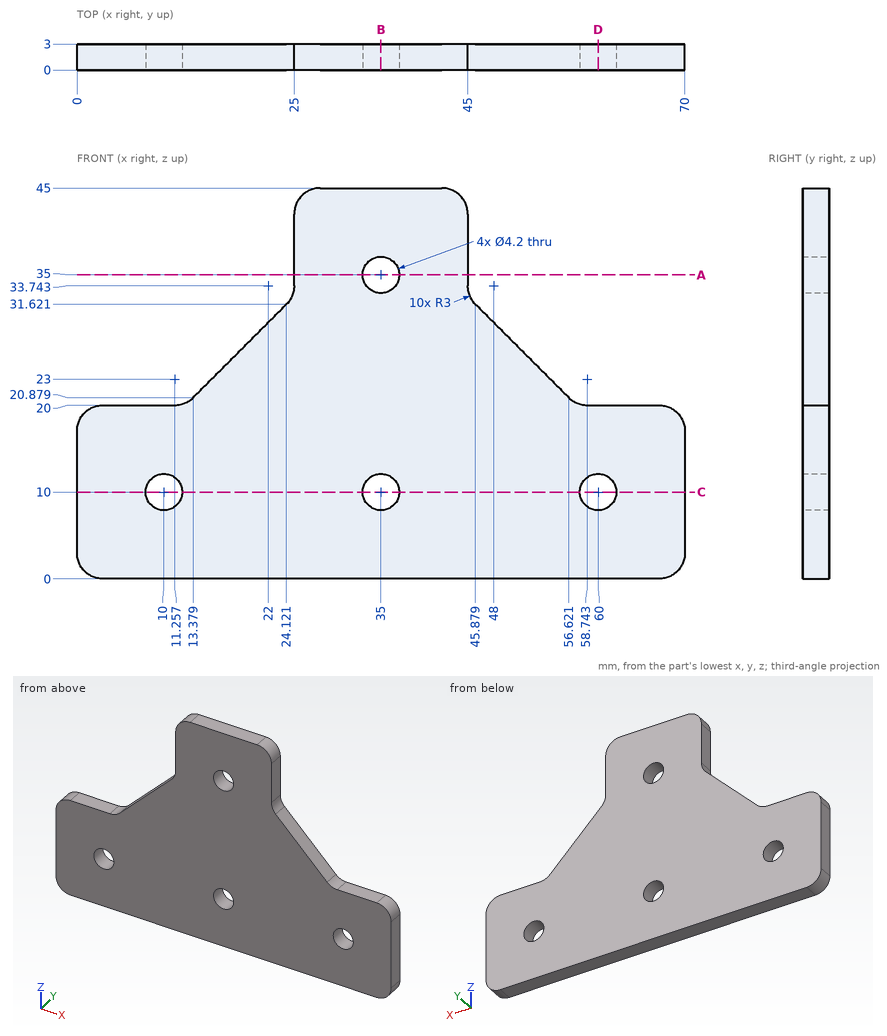
Design review of the part shown in the three views and the two pictorial views. Dimensions are in mm from the part's minimum x, y and z. Give positions to 0.01 mm unless a question says otherwise; leave off trailing zeros. Order: outer loops, then holes, each group sorted by start corner. A loop starts at its lowest first (then second) coordinate and runs counter-clockwise, first axis right, second up. Notation, with made-up numbers: M 16,62 L 69,62 A33 ccw 69,93 Z; hole C 46,-32.75 d10. An arc over 180 degrees is marked long. Answer in a Markdown table with one row per item. Add a question column.
(1) Consider section C-C on z = 10. State the section outline as (x, y) points, and give its area (3 significant figures).
(2) For pin 1 (2 mm diameter, centred on x = 55.5, z = 26, fed in from +Y); pin 2 (1 mm diameter, centred on y = 1, z = 26, fed in from -X); pin 3 (1.5 mm diameter, centred on y = 2, z = 39.5, fed in from +X); pin 4 (0.9 mm diameter, centred on x = 62, y = 1, fed in from +Z), all flat-tipped, find the tip position at first contact; note any pin that passes through.
(3) Consider section B-B on x = 35. State the section outline as (y, z) points.
(4) Wall thickness on probe 1 along X at (y, z) = (1.7, 10); probe 2 along X at (y, z) = (0.9, 35); probe 3 along Z at (x, y) = (66, 1): over which ranges is each line inside the solid? List them lowest first. Write a range as [from, to].
(5) Consider section A-A on z = 35. State the section outline as (x, y) points.
(6) Consider section D-D on x = 60. State the section outline as (y, z) points.
Evaluation:
| question | item | result |
|---|---|---|
| 1 | outline | M 0,0 L 7.9,0 L 7.9,3 L 0,3 Z; M 12.1,0 L 32.9,0 L 32.9,3 L 12.1,3 Z; M 37.1,0 L 57.9,0 L 57.9,3 L 37.1,3 Z; M 62.1,0 L 70,0 L 70,3 L 62.1,3 Z |
| 1 | area | 172 mm^2 |
| 2 | pin 1 | passes through |
| 2 | pin 2 | stops at x = 18 |
| 2 | pin 3 | stops at x = 45 |
| 2 | pin 4 | stops at z = 20 |
| 3 | outline | M 0,0 L 3,0 L 3,7.9 L 0,7.9 Z; M 0,12.1 L 3,12.1 L 3,32.9 L 0,32.9 Z; M 0,37.1 L 3,37.1 L 3,45 L 0,45 Z |
| 4 | probe 1 | x = [0, 7.9], [12.1, 32.9], [37.1, 57.9], [62.1, 70] |
| 4 | probe 2 | x = [25, 32.9], [37.1, 45] |
| 4 | probe 3 | z = [0, 20] |
| 5 | outline | M 25,0 L 32.9,0 L 32.9,3 L 25,3 Z; M 37.1,0 L 45,0 L 45,3 L 37.1,3 Z |
| 6 | outline | M 0,0 L 3,0 L 3,7.9 L 0,7.9 Z; M 0,12.1 L 3,12.1 L 3,20 L 0,20 Z |
